Work out the finished part from the listing and answer in its coordinate system (mm). A direction names the side the tool comes from. Round coordinates to 2 decimals unless told otherwise and drop trailing zeros. Loops run counter-clockwise (first coordinate to the right, second up) from the corner with the lowest first, then second, coordinate; pieces in that order, holes last. Notation, with made-up numbers: (63.5, 51) - (118.5, 51) arc R6 cw to (118.5, 60) - close; hole circle Ø6 at (88.5, -3.75). An arc over 180 degrees is marked (long way). Return JSON: item names as keys, results as strings.
from build123d import *

# Parameters (mm, degrees)
F0_W        = 53.7975355983
F0_H        = 80.8182843029
F0_H_2      = 16.7721658945
F0_H_3      = 21.6287262738
F0_H_4      = 0.8304491639
F0_H_5      = 12.1622607112
F1_DEPTH    = 127
F2_T        = 2.54
F2_T3_DEPTH = 132.08


# Not quite as in the source:
# - a shell that OpenCascade refuses in one call is made with other operations: the cavity is built on its own and cut out


with BuildPart() as f1:
    # F0 (on Front) → F1 (new body)
    with BuildSketch(Plane.XZ):
        with Locations((-143.1119032204, -0.0506583601)):
            Rectangle(F0_W, F0_H)
        with Locations((-143.1119032204, -48.8458834589)):
            Rectangle(F0_W, F0_H_2)
        with Locations((-143.1119032204, -68.046329543)):
            Rectangle(F0_W, F0_H_3)
        Polygon((-170.0106710196, 54.7638610005), (-170.0106710196, 40.3584837914), (-116.2131354213, 40.3584837914), (-74.950940907, 40.3584837914), (-43.6125695705, 40.3584837914), (-43.6125695705, 54.7638610005), (-116.2131354213, 54.7638610005), align=None)
        with Locations((-143.1119032204, -79.2759172618)):
            Rectangle(F0_W, F0_H_4)
        with Locations((-143.1119032204, 60.8449913561)):
            Rectangle(F0_W, F0_H_5)
        Polygon((-116.2131354213, -79.6911418438), (-170.0106710196, -79.6911418438), (-170.0106710196, -109.4150468707), (-9.6626672894, -109.4150468707), (-9.6626672894, -78.8606926799), (-13.8411177322, -78.8606926799), (-35.2556705475, -78.8606926799), (-35.2556705475, -79.6911418438), (-41.5233448148, -79.6911418438), (-41.5233448148, -78.8606926799), (-43.6125695705, -78.8606926799), (-43.6125695705, -79.6911418438), (-74.950940907, -79.6911418438), align=None)
        Polygon((-170.0106710196, 80.1929235458), (-170.0106710196, 66.9261217117), (-116.2131354213, 66.9261217117), (-43.6125695705, 66.9261217117), (-13.8411177322, 66.9261217117), (-9.6626672894, 66.9261217117), (-9.6626672894, 80.1929235458), align=None)
        Polygon((-13.8411177322, 54.7638610005), (-13.8411177322, 40.3584837914), (-13.8411177322, 6.9799921475), (-13.8411177322, -32.6986536384), (-13.8411177322, -78.8606926799), (-9.6626672894, -78.8606926799), (-9.6626672894, 66.9261217117), (-13.8411177322, 66.9261217117), align=None)
    extrude(amount=F1_DEPTH)

    # F2: shell of thickness 2.54, made by hand


with BuildPart() as f2_core1:
    # F2_t2: copy of F1
    add(f1.part)

    # the walls: a layer under each face that stays
    f2_faces = [f2_core1.faces().sort_by_distance(p)[0] for p in [
        (-79.9128524959, -63.5, 40.3584837914),
        (-43.6125695705, -63.5, 47.5611723959),
        (-79.9128524959, -63.5, 54.7638610005),
        (-116.2131354213, -63.5, 60.8449913561),
        (-65.0271265768, -63.5, 66.9261217117),
        (-13.8411177322, -63.5, -5.9672854841),
        (-24.5483941399, -63.5, -78.8606926799),
        (-35.2556705475, -63.5, -79.2759172618),
        (-38.3895076811, -63.5, -79.6911418438),
        (-41.5233448148, -63.5, -79.2759172618),
        (-42.5679571927, -63.5, -78.8606926799),
        (-43.6125695705, -63.5, -79.2759172618),
        (-79.9128524959, -63.5, -79.6911418438),
        (-116.2131354213, -63.5, -19.6663290262),
        (-89.8366691545, -63.5, 80.1929235458),
        (-170.0106710196, -63.5, -14.6110616624),
        (-89.8366691545, -63.5, -109.4150468707),
        (-9.6626672894, -63.5, -14.6110616624),
        (-143.2860037312, 0, -77.813718468),
    ]]
    thicken(f2_faces, amount=-F2_T, mode=Mode.SUBTRACT)

    # F2_s4 → F2_t3 (cut)
    with BuildSketch(Plane.XZ.offset(-2.54)):
        Polygon((-116.1877354213, 40.3330837914), (-116.2131354213, 42.8984837914), (-118.7531354213, 42.8984837914), (-118.7531354213, 40.3584837914), align=None)
        Polygon((-116.1877354213, 54.7892610005), (-116.2131354213, 52.2238610005), (-118.7531354213, 52.2238610005), (-118.7531354213, 54.7638610005), align=None)
        Polygon((-116.1877354213, 66.9007217117), (-118.7531354213, 66.9261217117), (-118.7531354213, 69.4661217117), (-116.2131354213, 69.4661217117), align=None)
        Polygon((-13.8665177322, 66.9007217117), (-13.8411177322, 69.4661217117), (-11.3011177322, 69.4661217117), (-11.3011177322, 66.9261217117), align=None)
        Polygon((-13.8665177322, -78.8352926799), (-11.3011177322, -78.8606926799), (-11.3011177322, -81.4006926799), (-13.8411177322, -81.4006926799), align=None)
        Polygon((-35.2810705475, -79.6657418438), (-32.7156705475, -79.6911418438), (-32.7156705475, -82.2311418438), (-35.2556705475, -82.2311418438), align=None)
        Polygon((-41.4979448148, -79.6657418438), (-41.5233448148, -82.2311418438), (-44.0633448148, -82.2311418438), (-44.0633448148, -79.6911418438), align=None)
        Polygon((-43.6379695705, -79.6657418438), (-41.0725695705, -79.6911418438), (-41.0725695705, -82.2311418438), (-43.6125695705, -82.2311418438), align=None)
        Polygon((-116.1877354213, -79.6657418438), (-116.2131354213, -82.2311418438), (-118.7531354213, -82.2311418438), (-118.7531354213, -79.6911418438), align=None)
    extrude(amount=F2_T3_DEPTH, mode=Mode.SUBTRACT)


with BuildPart() as f1_1:
    add(f1.part)

    # what is left inside the walls is the cavity
    f2_cavity = [f2_core1.part.solids().sort_by_distance(p)[0] for p in [
        (-167.445271, -85.513333, -14.611062),
    ]]
    add(f2_cavity, mode=Mode.SUBTRACT)


solid = f1_1.part
1) Section B-B (z = 49.5) is taken. Give the vertices of the cut face in (x, y).
Verdict:
{"outline": "(-170.01, -127) - (-167.47, -127) - (-167.47, -2.54) - (-46.15, -2.54) - (-46.15, -127) - (-43.61, -127) - (-43.61, 0) - (-170.01, 0) - close; (-13.84, -127) - (-9.66, -127) - (-9.66, 0) - (-13.84, 0) - close"}
2) A flat-ended cylindrical pin translates along its axis: pin 1 (2 mm diameter, centred on x = -81.5, z = -86, fed in from -Y). Find the tip coordinate at first contact, or state that the pin passes through.
Verdict:
{"pin 1": "stops at y = -2.54"}
3) Find the intervals of material crossed by L1, parallel to X at y = -104.5, z = 21.5; L2, parallel to X at y = -10, z = 51; L3, parallel to Z at x = -50, y = -13.5, in increasing order.
Verdict:
{"L1": "x = -170.01 to -167.47, -118.75 to -116.21, -13.84 to -9.66", "L2": "x = -170.01 to -167.47, -46.15 to -43.61, -13.84 to -9.66", "L3": "z = -109.42 to -106.88, -82.23 to -79.69, 40.36 to 42.9, 52.22 to 54.76, 66.93 to 69.47, 77.65 to 80.19"}
4) Determine the mould class of faces 1 (the flat face through (-170.011, -63, -13)), 2 (the flat face through (-43.613, -63, 47)), 3 (the flat face through (-13, -127, 14)) for opening direction X: pulls with the +X half, pulls with the -X half, needs draft (parallel to the pull), parting line crosses it, or undercut.
Verdict:
{"face 1": "pulls with the -X half", "face 2": "undercut", "face 3": "needs draft"}
5) A tool of negligible diameter and unlimited length cuts with its end or side. For faces 4 (the flat face through (-12.203, -64, 74)), 5 (the flat face through (-89, -63, 80.193)), 6 (the flat face through (-116.213, -63, -21)), from which of +Z, -Z, +X, -X, +Y, -Y can it reach the whole face along a straight path? Write none if from no direction.
Verdict:
{"face 4": "-Y", "face 5": "+Z, +X, -X, +Y, -Y", "face 6": "+Y, -Y"}
6) Section D-D (x = -134.5) is taken. Give the vertices of the cut face in (y, z), and give its area (3 significant figures).
Verdict:
{"outline": "(-127, -109.42) - (0, -109.42) - (0, 80.19) - (-127, 80.19) - (-127, 77.65) - (-2.54, 77.65) - (-2.54, -106.88) - (-127, -106.88) - close", "area": "1,110 mm2"}
7) Section C-C (x = -26) is taken. Give the vertices of the cut face in (y, z), and give its area (3 significant figures).
Verdict:
{"outline": "(-127, -109.42) - (0, -109.42) - (0, -78.86) - (-127, -78.86) - (-127, -81.4) - (-2.54, -81.4) - (-2.54, -106.88) - (-127, -106.88) - close; (-127, 66.93) - (0, 66.93) - (0, 80.19) - (-127, 80.19) - (-127, 77.65) - (-2.54, 77.65) - (-2.54, 69.47) - (-127, 69.47) - close", "area": "1,380 mm2"}
8) Section A-A (y = -19.5) is taken. Count the separate pieces of the cut face and the enclosed holes in it, and give its area (3 significant figures).
Verdict:
{"separate pieces": "1", "enclosed holes": "2", "area": "3,280 mm2"}
